Read the model definition and answer for the solid it produces. Units are mm, in the model's axes. A direction names the side the tool comes from. Round coordinates to 2 decimals unless told otherwise and drop trailing zeros. Order: outer loops, then holes, each group sorted by start corner. A loop starts at its lowest first (then second) coordinate and runs counter-clockwise, first axis right, second up. Notation, with made-up numbers: (35.5, 70) - (48.5, 70) arc R16 cw to (48.5, 100) - close; hole circle Ø5 at (89, 76.25). An arc over 180 degrees is marked (long way). Answer as a JSON object with one key per item and string values. Group by question number.
Q1. A cutting plane is placed at B-B on y = 0. Determine the outline of the cut face in (x, z), and give its area (3 significant figures).
Q2. The mould has two halves that part along Y. Classify faces 5 (the flat face through (30, 14, -20)), 6 (the cylindrical face through (-36, 0, -2)), 7 (the cylindrical face through (54.976, 1.099, -7.78)): pulls with the +Y half, pulls with the -Y half, needs draft (parallel to the pull), parting line crosses it, or undercut.
Q3. Given pin 1 Ø6 at (x, y) = (-18, 2.5) entering from -Z; pin 2 Ø3 at (x, z) = (-26, -2) entering from +Y; pin 3 Ø19 at (x, y) = (-15.5, 1) entering from -Z, each flat-ended and moving along its own axis, determine where each tip first touches the part or whether it passes through.
Q4. A cutting plane is placed at A-A on z = -17. Determine the outline of the cut face in (x, y).
Q5. A cutting plane is placed at C-C on x = 3.5. Determine the outline of the cut face in (y, z), and give its area (3 significant figures).
Q6. A tool of negligible diameter and unlimited length cuts with its end or side. For faces 1 (the flat face through (-1, 0, 6)), 2 (the cylindrical face through (-42, 0, -2)), 3 (the flat face through (46, 6, -17)), 4 (the flat face through (-12, 11, 0)), from which of +Z, -Z, +X, -X, +Y, -Y can it reach the whole face along a straight path? Write none if from no direction.
Q7. Consider line 1 (X direction, y = 0, z = -13); line 2 (Y direction, x = -7, z = 10); line 3 (Y direction, x = -19, z = -3). Determine where each line is inside the solid, lowest interval first.
Q8. A cutting plane is placed at D-D on z = -5.5. Determine the outline of the cut face in (x, y).
```python
from build123d import *

# Parameters (mm, degrees)
BOSS_EXTRUDE1_DEPTH = 12
SKETCH2_W           = 115.368929346
SKETCH2_H           = 20
CUT_EXTRUDE1_DEPTH  = 6
BOSS_EXTRUDE2_START = 20
SKETCH3_R           = 25
SKETCH3_R_2         = 10
BOSS_EXTRUDE2_DEPTH = 20
SKETCH4_W           = 50
SKETCH4_H           = 12
CUT_EXTRUDE2_DEPTH  = 6
BOSS_EXTRUDE3_DEPTH = 4


with BuildPart() as part:
    # Sketch1 → Boss-Extrude1 (new body)
    with BuildSketch(Plane.XY):
        with BuildLine():
            Line((30, -25), (-30, -25))
            ThreePointArc((-30, -25), (-55, 0), (-30, 25))
            Line((-30, 25), (30, 25))
            ThreePointArc((30, 25), (55, 0), (30, -25))
        make_face()
    extrude(amount=BOSS_EXTRUDE1_DEPTH)

    # Sketch2 → Cut-Extrude1 (cut)
    with BuildSketch(Plane.XY.offset(12)):
        Rectangle(SKETCH2_W, SKETCH2_H)
    extrude(amount=-CUT_EXTRUDE1_DEPTH, mode=Mode.SUBTRACT)

    # Sketch3 → Boss-Extrude2 (add)
    with BuildSketch(Plane(origin=(0, 0, 0), x_dir=(-1, 0, 0), z_dir=(0, 0, -1)).offset(BOSS_EXTRUDE2_START)):
        with Locations((-30, 0)):
            Circle(SKETCH3_R)
        with Locations((-30, 0)):
            Circle(SKETCH3_R_2, mode=Mode.SUBTRACT)
    extrude(amount=-BOSS_EXTRUDE2_DEPTH)

    # Sketch4 → Cut-Extrude2 (cut)
    with BuildSketch(Plane(origin=(0, 0, -20), x_dir=(-1, 0, 0), z_dir=(0, 0, -1))):
        with Locations((-30, 0)):
            Rectangle(SKETCH4_W, SKETCH4_H)
    extrude(amount=-CUT_EXTRUDE2_DEPTH, mode=Mode.SUBTRACT)

    # Sketch5 → Boss-Extrude3 (add)
    with BuildSketch(Plane(origin=(0, 0, 0), x_dir=(-1, 0, 0), z_dir=(0, 0, -1))):
        with BuildLine():
            Line((18, 12), (30, 12))
            ThreePointArc((30, 12), (42, 0), (30, -12))
            Line((30, -12), (18, -12))
            ThreePointArc((18, -12), (6, 0), (18, 12))
        make_face()
        with BuildLine():
            Line((18, 6), (30, 6))
            ThreePointArc((30, 6), (36, 0), (30, -6))
            Line((30, -6), (18, -6))
            ThreePointArc((18, -6), (12, 0), (18, 6))
        make_face(mode=Mode.SUBTRACT)
    extrude(amount=BOSS_EXTRUDE3_DEPTH)


solid = part.part
```
Result set:
{
 "1": {"outline": "(-55, 0) - (-42, 0) - (-42, -4) - (-36, -4) - (-36, 0) - (-12, 0) - (-12, -4) - (-6, -4) - (-6, 0) - (5, 0) - (5, -14) - (20, -14) - (20, 0) - (40, 0) - (40, -14) - (55, -14) - (55, 6) - (-55, 6) - close", "area": "1,130 mm²"},
 "2": {"face 5": "needs draft", "face 6": "undercut", "face 7": "parting line crosses it"},
 "3": {"pin 1": "stops at z = 0", "pin 2": "stops at y = 12", "pin 3": "stops at z = -4"},
 "4": {"outline": "(5.73, -6) arc R25 ccw to (54.27, -6) - (38, -6) arc R10 cw to (22, -6) - close; (5.73, 6) - (22, 6) arc R10 cw to (38, 6) - (54.27, 6) arc R25 ccw to start"},
 "5": {"outline": "(-25, 0) - (25, 0) - (25, 12) - (10, 12) - (10, 6) - (-10, 6) - (-10, 12) - (-25, 12) - close", "area": "480 mm²"},
 "6": {"face 1": "+Z, +X, -X", "face 2": "-Z, -X", "face 3": "-Z, +X, -X", "face 4": "-Z"},
 "7": {"line 1": "x = 5 to 20, 40 to 55", "line 2": "y = -25 to -10, 10 to 25", "line 3": "y = -12 to -6, 6 to 12"},
 "8": {"outline": "circle Ø50 at (30, 0); hole circle Ø20 at (30, 0)"}
}
